Read the model definition and answer for the solid it produces. Units are mm, in the model's axes. A direction names the side the tool comes from. Coordinates: 2 decimals unless noted, no trailing zeros. Write item = value, one per line. Start each with the question number.
1) For a pull along Z with two mould halves and no side action, classify faces 5 (the face through (-10, 0, -24)), 6 (the face through (36, 13, 50)), 7 (the face through (37.292, 13.286, 49.493)), 8 (the face through (-8.94, -40.27, 41.49)) as released by +Z, released by -Z, zero draft, split by the parting line, or undercut.
2) Flat-ended cylindrical pins translate along their axes: pin 1 Ø1.5 at (y, z) = (13, -22.5) entering from -X; pin 2 Ø2.5 at (x, y) = (0, -38.5) entering from +Z; pin 3 Ø1 at (x, y) = (17, 12.5) entering from +Z. Find the tip coordinate at first contact, or state that the pin passes through.
3) Find the intervals of material crossed by line 1 along Z through (x, y) = (6.5, -27.5); line 2 along Y through (x, z) = (1, -41); line 3 along X through (y, z) = (0, -25), in increasing order. Write a range as from..to.
4) A tool of negligible diameter and unlimited length cuts with its end or side. For faces 1 (the face through (-29.11, 26.7, 20.49)), 2 (the face through (16, 37, 50)), 3 (the face through (-20, 0, -42)), 4 (the face through (26.772, -28.654, 49.493)), from which of +Z, -Z, +X, -X, +Y, -Y can it reach the whole face along a straight path? Write none if from no direction.
from build123d import *

# Parameters (mm, degrees)
SKETCH2_R           = 39.5
BOSS_EXTRUDE1_DEPTH = 1
SKETCH4_R           = 41.25
BOSS_EXTRUDE2_DEPTH = 1
SKETCH5_R           = 42
BOSS_EXTRUDE3_DEPTH = 7
SKETCH6_R           = 35
BOSS_EXTRUDE4_DEPTH = 3
SKETCH7_R           = 2.25
SKETCH7_R_2         = 1.5
BOSS_EXTRUDE5_DEPTH = 1
CIRPATTERN1_COUNT   = 16
SKETCH8_W           = 20
SKETCH8_H           = 40
BOSS_EXTRUDE6_DEPTH = 42
SKETCH9_R           = 20
BOSS_EXTRUDE7_DEPTH = 20
SKETCH10_R          = 10
BOSS_EXTRUDE8_DEPTH = 10
SKETCH11_R          = 10
BOSS_EXTRUDE9_DEPTH = 10


with BuildPart() as part:
    # Sketch1 → Revolve1 (revolve)
    with BuildSketch(Plane(origin=(0, 0, 0), x_dir=(1, 0, 0), z_dir=(0, 1, 0))):
        with BuildLine():
            Line((0, 0), (0, -20))
            Line((0, -20), (-42, -20))
            ThreePointArc((-42, -20), (-39.360679775, -8.819660113), (-32, 0))
            Line((-32, 0), (0, 0))
        make_face()
    revolve(axis=Axis((0, 0, 0), (0, 0, 1)))

    # Sketch2 → Boss-Extrude1 (add)
    with BuildSketch(Plane.XY.offset(20)):
        Circle(SKETCH2_R)
    extrude(amount=BOSS_EXTRUDE1_DEPTH)

    # Sketch3 → Revolve2 (revolve)
    with BuildSketch(Plane(origin=(0, 0, 0), x_dir=(1, 0, 0), z_dir=(0, 1, 0))):
        with BuildLine():
            Line((0, -21), (-40, -21))
            ThreePointArc((-40, -21), (-41.376973739, -31), (-40, -41))
            Line((-40, -41), (0, -41))
            Line((0, -41), (0, -21))
        make_face()
    revolve(axis=Axis((0, 0, 21), (0, 0, 1)))

    # Sketch4 → Boss-Extrude2 (add)
    with BuildSketch(Plane.XY.offset(41)):
        Circle(SKETCH4_R)
    extrude(amount=BOSS_EXTRUDE2_DEPTH)

    # Sketch5 → Boss-Extrude3 (add)
    with BuildSketch(Plane.XY.offset(42)):
        Circle(SKETCH5_R)
    extrude(amount=BOSS_EXTRUDE3_DEPTH)

    # Sketch6 → Boss-Extrude4 (add)
    with BuildSketch(Plane.XY.offset(49)):
        Circle(SKETCH6_R)
    extrude(amount=BOSS_EXTRUDE4_DEPTH)

    # Sketch7 → Boss-Extrude5 (add)
    with BuildSketch(Plane.XY.offset(49)):
        with Locations((38.5, 0)):
            Circle(SKETCH7_R)
        with Locations((38.5, 0)):
            Circle(SKETCH7_R_2, mode=Mode.SUBTRACT)
    boss_extrude5 = extrude(amount=BOSS_EXTRUDE5_DEPTH)

    # CirPattern1: Boss-Extrude5 ×16 about axis
    cirpattern1_axis = Axis((0, 0, 0), (0, 0, 1))
    for i in range(1, CIRPATTERN1_COUNT):
        add(boss_extrude5.rotate(cirpattern1_axis, i * 360 / CIRPATTERN1_COUNT))

    # Sketch8 → Boss-Extrude6 (add)
    with BuildSketch(Plane(origin=(0, 0, 0), x_dir=(-1, 0, 0), z_dir=(0, 0, -1))):
        Rectangle(SKETCH8_W, SKETCH8_H)
    extrude(amount=BOSS_EXTRUDE6_DEPTH)

    # Sketch9 → Boss-Extrude7 (add)
    with BuildSketch(Plane.ZY.offset(10)):
        with Locations((-42, 0)):
            Circle(SKETCH9_R)
    extrude(amount=-BOSS_EXTRUDE7_DEPTH)

    # Sketch10 → Boss-Extrude8 (add)
    with BuildSketch(Plane.ZY.offset(10)):
        with Locations(Location((-42, 0, 0), (0, 0, 90))):
            Circle(SKETCH10_R)
    extrude(amount=BOSS_EXTRUDE8_DEPTH)

    # Sketch11 → Boss-Extrude9 (add)
    with BuildSketch(Plane.XY.offset(52)):
        Circle(SKETCH11_R)
    extrude(amount=BOSS_EXTRUDE9_DEPTH)


solid = part.part
Answer key:
q1.face_5 = undercut
q1.face_6 = released by +Z
q1.face_7 = zero draft
q1.face_8 = undercut
q2.pin_1 = -10
q2.pin_2 = 49
q2.pin_3 = 52
q3.line_1 = 0..52
q3.line_2 = -20..20
q3.line_3 = -10..10
q4.face_1 = none
q4.face_2 = +Z, +X, +Y
q4.face_3 = -Z, -X, +Y, -Y
q4.face_4 = +Z
